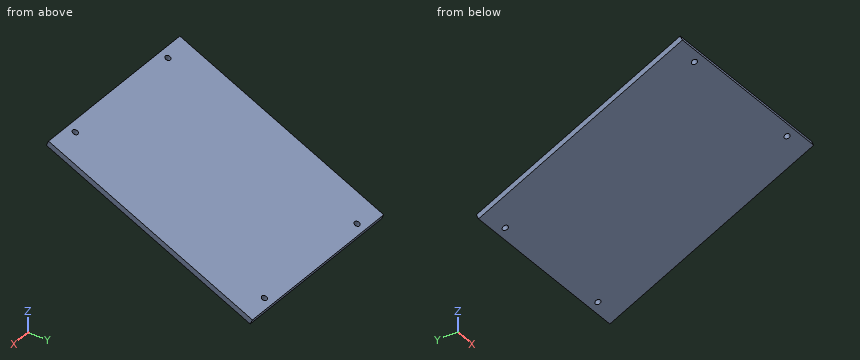
```python
from build123d import *

# Parameters (mm, degrees)
BOSS_EXTRUDE1_DEPTH         = 215.9
F_1_4_0_25_DIAMETER_HOLE1_D = 6.35


with BuildPart() as part:
    # Sketch1 → Boss-Extrude1 (new body)
    with BuildSketch(Plane(origin=(0, 0, 0), x_dir=(0, 0, -1), z_dir=(1, 0, 0))):
        Polygon((0, 0), (111.727575693, 237.838071514), (105.980151385, 240.538), (-5.747424307, 2.699928486), align=None)
    extrude(amount=BOSS_EXTRUDE1_DEPTH)

    # 1/4 (0.25) Diameter Hole1 (through all)
    with Locations(Plane(origin=(0, 2.699928486, 5.747424307), x_dir=(1, 0, 0), z_dir=(0, 0.425185588, 0.90510619))):
        with Locations((31.75, 253.248665788), (184.15, 253.248665788), (184.15, 9.525), (31.75, 9.525)):
            Hole(F_1_4_0_25_DIAMETER_HOLE1_D / 2)


solid = part.part
```
Can you work these out from the model? Positions are in its coordinate system, mm. Coordinates: 2 decimals unless noted, no trailing zeros. Write each loop counter-clockwise with the first axis right and the second up, starting at its lowest first coordinate (ties: lowest second). Pieces come first, ordered by that corner, then holes. Notation, with made-up numbers: M -7,-36 L 42,-36 A10 cw 42,-19 Z; hole C -6,3.25 d4. An arc over 180 degrees is marked long. Write item = value, one per line. Start each with the question number.
Q1. If we section it at A-A, the plane x = 199.5: Write out the boundary of the cut face in (y, z).
Q2. I'm going to push flat-ended pins straight in: pin 1 (3 mm diameter, centred on x = 25, y = 157, fed in from +Z); pin 2 (4 mm diameter, centred on x = 130, y = 124, fed in from +Z); pin 3 (12 mm diameter, centred on x = 31.5, y = 54.5, fed in from +Z). Where does each tip first touch, or does it pass through?
Q3. If I drill on L1, parallel to Z at x = 9, y = 54.5; L2, parallel to Z at x = 198, y = 171.5; L3, parallel to Y at x = 56, z = -61.5, over which ranges is the centre line in solid material (lowest first)? Write a range as [from, to].
Q4. If we section it at B-B, the plane y = 162: Write out the boundary of the cut face in (x, z).
Check sheet entries:
q1.outline = M 0,0 L 237.84,-111.73 L 240.54,-105.98 L 2.7,5.75 Z
q2.pin_1 = -66.03
q2.pin_2 = -50.3
q2.pin_3 = -15.77
q3.L1 = [-25.6, -18.59]
q3.L2 = [-80.56, -73.55]
q3.L3 = [130.92, 145.85]
q4.outline = M 0,-76.1 L 215.9,-76.1 L 215.9,-69.09 L 0,-69.09 Z
